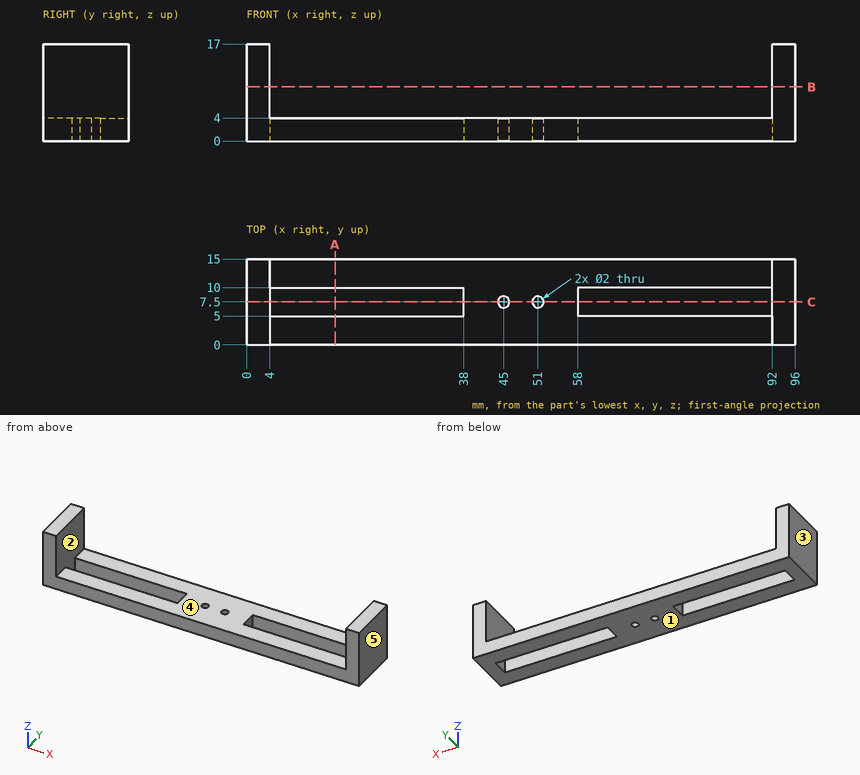
Design review of the part shown in the three views and the two pictorial views. Dimensions are in mm from the part's minimum x, y and z. A direction names the side the tool comes from. Round coordinates to 2 decimals unless told otherwise and drop trailing zeros. Order: outer loops, then holes, each group sorted by start corner. A loop starts at its lowest first (then second) coordinate and runs counter-clockwise, first axis right, second up.
Item 1: Add section A-A, the plane x = 15.5. State the section outline as (y, z) points.
Working result:
outline: (0, 0) - (5, 0) - (5, 4) - (0, 4) - close; (10, 0) - (15, 0) - (15, 4) - (10, 4) - close
Item 2: Add section C-C, the plane y = 7.5. State the section outline as (x, z) points.
Working result:
outline: (0, 0) - (4, 0) - (4, 17) - (0, 17) - close; (38, 0) - (44, 0) - (44, 4) - (38, 4) - close; (46, 0) - (50, 0) - (50, 4) - (46, 4) - close; (52, 0) - (58, 0) - (58, 4) - (52, 4) - close; (92, 0) - (96, 0) - (96, 17) - (92, 17) - close
Item 3: Machinability: for the marked faces 4 and 5, which of the approach directions +Z, -Z, +X, -X, +Y, -Y give a long, thin tool a straight path to every point of the face, cutting with its end or side? Answer none if there is none.
Working result:
face 4: +Z, +Y, -Y
face 5: +Z, -Z, +X, +Y, -Y
Item 4: To check wall thickness, follow probe 1 along X at (y, z) = (7.5, 2.7); probe 2 along X at (y, z) = (13.5, 14); probe 3 along Y at (x, z) = (51, 1.7). State the ranges of each line that lie inside material, in increasing order.
Working result:
probe 1: x = 0 to 4, 38 to 44, 46 to 50, 52 to 58, 92 to 96
probe 2: x = 0 to 4, 92 to 96
probe 3: y = 0 to 6.5, 8.5 to 15
Item 5: Add section B-B, the plane z = 9.5. State the section outline as (x, y) points.
Working result:
outline: (0, 0) - (4, 0) - (4, 15) - (0, 15) - close; (92, 0) - (96, 0) - (96, 15) - (92, 15) - close
Item 6: For pin 1 (7.5 mm diameter, centred on x = 39.5, y = 10, fed in from +Z), flat-tipped, find the tip position at first contact; note if it passes through.
Working result:
pin 1: stops at z = 4
Item 7: Draft analysis for pull direction X (two halves, no side actions). For the marked faces 1, 2 and 3, state which applies: released by +X, released by -X, zero draft, split by the parting line, or undercut.
Working result:
face 1: zero draft
face 2: undercut
face 3: released by -X
